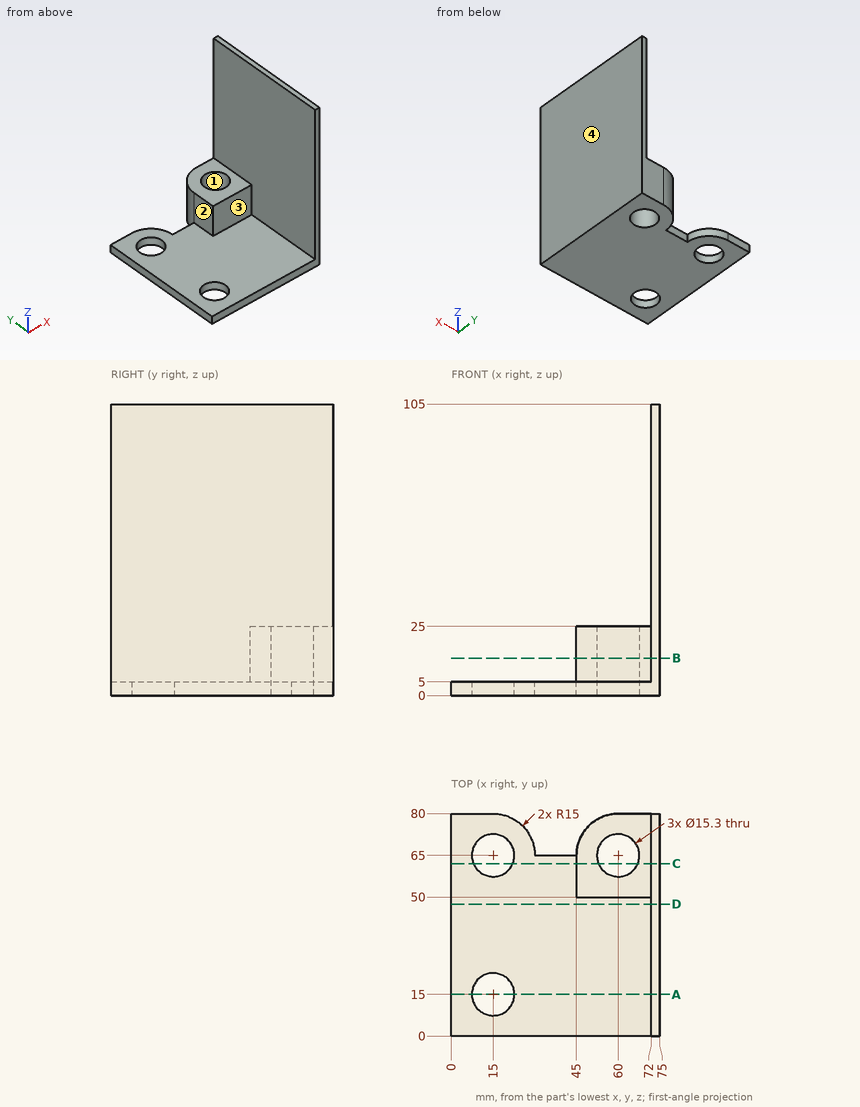
Here's the drawing with two shaded views (mm, measured from the low corner). I have some questions. Coordinates: 2 decimals unless noted, no trailing zeros. Order: outer loops, then holes, each group sorted by start corner. A loop starts at its lowest first (then second) coordinate and runs counter-clockwise, first axis right, second up.
Item 1: If we section it at C-C on y = 62: List the corners of the cut face in (x, z) for me, plus the area to 3 significant figures.
Result sheet:
outline: (0, 0) - (7.96, 0) - (7.96, 5) - (0, 5) - close; (22.04, 0) - (52.96, 0) - (52.96, 25) - (45, 25) - (45, 5) - (22.04, 5) - close; (67.04, 0) - (75, 0) - (75, 105) - (72, 105) - (72, 25) - (67.04, 25) - close
area: 793 mm2
Item 2: If we section it at B-B on z = 13.5: List the corners of the cut face in (x, y) for me.
Result sheet:
outline: (45, 50) - (72, 50) - (72, 0) - (75, 0) - (75, 80) - (60, 80) arc R15 ccw to (45, 65) - close; hole circle Ø15.3 at (60, 65)
Item 3: If we mould it in two halves opening along X, with no side actions, what happens to the marked faces 1, 2, 3 and 4? For each: +X half, -X half, draft (parallel to the pull), parting line (faces both ways), or undercut.
Result sheet:
face 1: undercut
face 2: -X half
face 3: draft
face 4: +X half
Item 4: I need wall thicknesses on line 1 (Y direction, x = 15, z = 1.6); line 2 (Y direction, x = 60, z = 12.75); line 3 (Z direction, x = 65, y = 33). Which ranges of each line are inside material? Lowest first, please.
Result sheet:
line 1: y = 0 to 7.35, 22.65 to 57.35, 72.65 to 80
line 2: y = 50 to 57.35, 72.65 to 80
line 3: z = 0 to 5
Item 5: For P1, Ø1.5, axis at x = 38, z = 2, coming from the +Y side; P2, Ø7.5, axis at y = 58.5, z = 13, coming from the -X side; P3, Ø13.5, axis at x = 58, y = 58, coming from the +Z side, each with a flat end and sliding along its axis, tell me the tip position at first contact or that it passes through.
Result sheet:
P1: stops at y = 65
P2: stops at x = 45
P3: stops at z = 25
Item 6: If we section it at D-D on y = 47.5: List the corners of the cut face in (x, z) for me, plus the area to 3 significant figures.
Result sheet:
outline: (0, 0) - (75, 0) - (75, 105) - (72, 105) - (72, 5) - (0, 5) - close
area: 675 mm2
Item 7: If we section it at A-A on y = 15: List the corners of the cut face in (x, z) for me.
Result sheet:
outline: (0, 0) - (7.35, 0) - (7.35, 5) - (0, 5) - close; (22.65, 0) - (75, 0) - (75, 105) - (72, 105) - (72, 5) - (22.65, 5) - close
